```python
from build123d import *

# Parameters (mm, degrees)
F0_W      = 152.3159295321
F0_H      = 151.994921267
F1_DEPTH  = 25.4
F2_R      = 5.08
F3_R      = 5.08
F4_DEPTH  = 25.4
F5_SIZE   = 5.08
F6_DEPTH  = 25.4
F7_SIZE   = 5.08
F8_DEPTH  = 25.4
F9_R      = 5.08
F10_DEPTH = 25.4
F11_R     = 5.08
F12_DEPTH = 25.4
F13_SIZE  = 5.08
F14_DEPTH = 25.4
F15_SIZE  = 5.08
F16_DEPTH = 25.4
F17_R     = 5.08
F18_DEPTH = 25.4
F19_R     = 5.08


with BuildPart() as f1:
    # F0 (on Top) → F1 (new body)
    with BuildSketch(Plane.XY):
        with Locations((0.3210008144, -0.3210045397)):
            Rectangle(F0_W, F0_H)
    extrude(amount=F1_DEPTH)

    # F2
    f2_edges = [f1.edges().sort_by_distance(p)[0] for p in [
        (0.321001, 75.676456, 25.4),
        (-75.836964, -0.321005, 25.4),
        (0.321001, -76.318465, 25.4),
        (76.478966, -0.321005, 25.4),
    ]]
    fillet(f2_edges, radius=F2_R)

    # F3
    f3_edges = [f1.edges().sort_by_distance(p)[0] for p in [
        (0.321001, 75.676456, 0),
        (-75.836964, -0.321005, 0),
        (0.321001, -76.318465, 0),
        (76.478966, -0.321005, 0),
    ]]
    fillet(f3_edges, radius=F3_R)

    # F4 (add): a face of the model
    f4_faces = [f1.faces().sort_by_distance(p)[0] for p in [
        (0.3210008144, -0.3210045397, 0),
    ]]
    extrude(f4_faces, amount=F4_DEPTH)

    # F5
    f5_edges = [f1.edges().sort_by_distance(p)[0] for p in [
        (0.321001, 70.596456, -25.4),
        (71.398966, -0.321005, -25.4),
        (-70.756964, -0.321005, -25.4),
        (0.321001, -71.238465, -25.4),
    ]]
    chamfer(f5_edges, length=F5_SIZE)

    # F6 (add): a face of the model
    f6_faces = [f1.faces().sort_by_distance(p)[0] for p in [
        (0.3210008144, -0.3210045397, 25.4),
    ]]
    extrude(f6_faces, amount=F6_DEPTH)

    # F7
    f7_edges = [f1.edges().sort_by_distance(p)[0] for p in [
        (0.321001, 70.596456, 50.8),
        (71.398966, -0.321005, 50.8),
        (-70.756964, -0.321005, 50.8),
        (0.321001, -71.238465, 50.8),
    ]]
    chamfer(f7_edges, length=F7_SIZE)

    # F8 (add): a face of the model
    f8_faces = [f1.faces().sort_by_distance(p)[0] for p in [
        (0.3210008144, -0.3210045397, 50.8),
    ]]
    extrude(f8_faces, amount=F8_DEPTH)

    # F9
    f9_edges = [f1.edges().sort_by_distance(p)[0] for p in [
        (0.321001, 65.516456, 76.2),
        (66.318966, -0.321005, 76.2),
        (-65.676964, -0.321005, 76.2),
        (0.321001, -66.158465, 76.2),
    ]]
    fillet(f9_edges, radius=F9_R)

    # F10 (add): a face of the model
    f10_faces = [f1.faces().sort_by_distance(p)[0] for p in [
        (0.3210008144, -0.3210045397, -25.4),
    ]]
    extrude(f10_faces, amount=F10_DEPTH)

    # F11
    f11_edges = [f1.edges().sort_by_distance(p)[0] for p in [
        (0.321001, 65.516456, -50.8),
        (66.318966, -0.321005, -50.8),
        (-65.676964, -0.321005, -50.8),
        (0.321001, -66.158465, -50.8),
    ]]
    fillet(f11_edges, radius=F11_R)

    # F12 (add): a face of the model
    f12_faces = [f1.faces().sort_by_distance(p)[0] for p in [
        (0.3210008144, -0.3210045397, -50.8),
    ]]
    extrude(f12_faces, amount=F12_DEPTH)

    # F13
    f13_edges = [f1.edges().sort_by_distance(p)[0] for p in [
        (0.321001, 60.436456, -76.2),
        (61.238966, -0.321005, -76.2),
        (-60.596964, -0.321005, -76.2),
        (0.321001, -61.078465, -76.2),
    ]]
    chamfer(f13_edges, length=F13_SIZE)

    # F14 (add): a face of the model
    f14_faces = [f1.faces().sort_by_distance(p)[0] for p in [
        (0.3210008144, -0.3210045397, 76.2),
    ]]
    extrude(f14_faces, amount=F14_DEPTH)

    # F15
    f15_edges = [f1.edges().sort_by_distance(p)[0] for p in [
        (0.321001, 60.436456, 101.6),
        (61.238966, -0.321005, 101.6),
        (-60.596964, -0.321005, 101.6),
        (0.321001, -61.078465, 101.6),
    ]]
    chamfer(f15_edges, length=F15_SIZE)

    # F16 (add): a face of the model
    f16_faces = [f1.faces().sort_by_distance(p)[0] for p in [
        (0.3210008144, -0.3210045397, 101.6),
    ]]
    extrude(f16_faces, amount=F16_DEPTH)

    # F17
    f17_edges = [f1.edges().sort_by_distance(p)[0] for p in [
        (0.321001, 55.356456, 127),
        (56.158966, -0.321005, 127),
        (-55.516964, -0.321005, 127),
        (0.321001, -55.998465, 127),
    ]]
    fillet(f17_edges, radius=F17_R)

    # F18 (add): a face of the model
    f18_faces = [f1.faces().sort_by_distance(p)[0] for p in [
        (0.3210008144, -0.3210045397, -76.2),
    ]]
    extrude(f18_faces, amount=F18_DEPTH)

    # F19
    f19_edges = [f1.edges().sort_by_distance(p)[0] for p in [
        (0.321001, 55.356456, -101.6),
        (56.158966, -0.321005, -101.6),
        (-55.516964, -0.321005, -101.6),
        (0.321001, -55.998465, -101.6),
    ]]
    fillet(f19_edges, radius=F19_R)


solid = f1.part
```
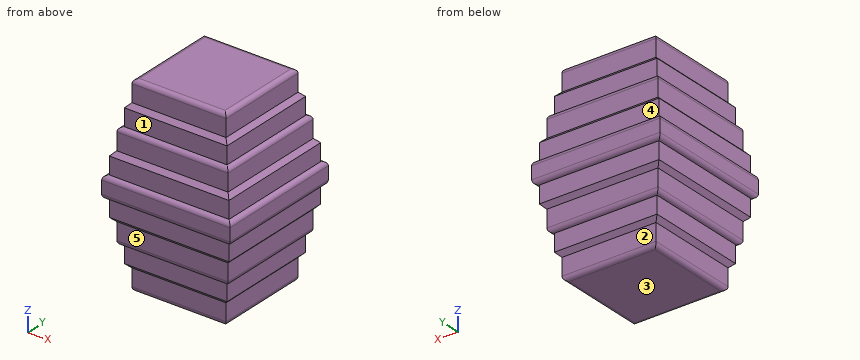
The model under review builds one solid part; all positions refer to its coordinate system, in mm. Face numbers are marked on the shaded views. A direction names the side the tool comes from. Give positions to 0.01 mm unless a question says otherwise; leave off trailing zeros. Loops run counter-clockwise (first coordinate to the right, second up) from the corner with the lowest first, then second, coordinate; pieces in that order, holes last. Notation, with made-up numbers: (1.5, 87.5) -> (29.5, 87.5) arc R26 ccw to (29.5, 112.5) -> close; hole circle Ø11 at (64.25, -16). An arc over 180 degrees is marked (long way). Use CSV: the item, a comma, the result in double quotes.
1. To check wall thickness, follow probe 1 along Y at (x, z) = (5.5, -46); probe 2 along Y at (x, z) = (51, -52); probe 3 along X at (y, z) = (9.5, 52). State the ranges of each line that lie inside material, in increasing order. Write a range as from..to.
Result:
probe 1,"y = -66.15..65.51"
probe 2,"y = -61.08..60.44"
probe 3,"x = -65.68..66.32"
2. Machinability: for the marked faces 1, 2, 3, 4 and 5, which of the approach directions +Z, -Z, +X, -X, +Y, -Y give a long, thin tool a straight path to every point of the face, cutting with its end or side? Answer none if there is none.
Result:
face 1,"+Z, +X, -X, -Y"
face 2,"-Z, +X, -X, +Y"
face 3,"-Z, +X, -X, +Y, -Y"
face 4,"+Z, +X, -X, +Y"
face 5,"-Z, +X, -X, -Y"
3. For P1, Ø16.5, axis at y = 19, z = 108, coming from the -X side; P2, Ø16.5, axis at x = 3, z = 89.5, coming from the -Y side; P3, Ø12, axis at y = -1.5, z = 96.5, coming from the -X side, all flat-tipped, find the tip position at first contact; note any pin that passes through.
Result:
P1,"stops at x = -57.37"
P2,"stops at y = -61.08"
P3,"stops at x = -60.6"
4. Consider section B-B, the plane z = 79. Write out the cut boundary in (x, y), then the cut area to 3 significant figures.
Result:
outline,"(-60.6, -61.08) -> (61.24, -61.08) -> (61.24, 60.44) -> (-60.6, 60.44) -> close"
area,"14,800 mm²"
5. Consider section A-A, the plane z = 36. Write out the cut boundary in (x, y).
Result:
outline,"(-70.76, -71.24) -> (71.4, -71.24) -> (71.4, 70.6) -> (-70.76, 70.6) -> close"
